Source: CAD feature listing. Evaluate the final solid. Frame: model axes, mm. A direction names the side the tool comes from. Give positions to 0.01 mm unless a question says otherwise; leave off trailing zeros. Write each loop counter-clockwise with the first axis right and the second up, starting at its lowest first coordinate (ties: lowest second). Pieces come first, ordered by that corner, then holes. Notation, with made-up numbers: (-38.75, 72.25) -> (-18.75, 72.25) arc R10 ccw to (-18.75, 91.25) -> close; hole circle Ø10 at (33, -38). An arc over 180 degrees is marked (long way). Answer as a JSON object with one key per item and string values. Group by question number.
Item 1: Section query D-D on y = 3.25. Return the cut outline in (x, z).
Item 2: Section query C-C on x = 0. Return the cut outline in (y, z).
Item 3: Section query A-A on z = 6.25. Return the cut outline in (x, y).
Item 4: Section query B-B on z = 1.75. Return the cut outline in (x, y).
Item 5: First-contact query: pin 1 Ø1 at (y, z) = (3, 6) entering from -X; pin 2 Ø1 at (x, z) = (2.5, 6.5) entering from +Y; pin 3 Ø0.8 at (x, y) = (-5.5, 2.5) entering from +Z. Flat tips, straight axial feed; report the tip coordinate or a pass-through.
Item 6: Ray query, probe 1 along X at (y, z) = (3.75, 5); probe 2 along X at (y, z) = (-3.25, 0.75); probe 3 along Y at (x, z) = (-2.25, 2.5). Return the intervals inside material, ascending. Write a range as from..to.
Item 7: Access query for faces 1 (the face through (3, -4, 6)), 2 (the face through (3, 1.5, 6)), 3 (the face through (5.5, 0.1, 2)). Directions: +Z, -Z, +X, -X, +Y, -Y. A direction counts if a zero-diameter tool reaches every point of the face in a straight line with its end or side. Return the directions, or none.
Item 8: Pull-direction query (Y, two-part tool) for faces 4 (the face through (5, -0.1, 3.6)), 5 (the face through (0, 10, 2)), 6 (the face through (0, 0, 3)); classes: pulls with the +Y half, pulls with the -Y half, needs draft (parallel to the pull), parting line crosses it, or undercut.
Autodesk Inventor part; units mm, degrees
ref_plane "YZ Plane" through (0, 0, 0) normal (1, 0, 0) x (0, 1, 0)
ref_plane "XZ Plane" through (0, 0, 0) normal (0, 1, 0) x (-1, 0, 0)
ref_plane "XY Plane" through (0, 0, 0) normal (0, 0, 1) x (1, 0, 0)
sketch "Sketch1" plane through (0, 0, 0) normal (0, 0, 1) x (1, 0, 0)
  line L0 (-6, -10) -> (6, -10)
  line L1 (6, -10) -> (6, 10)
  line L2 (6, 10) -> (-6, 10)
  line L3 (-6, 10) -> (-6, -10)
  line L4 (-6, -10) -> (6, 10) construction
  line L5 (6, -10) -> (-6, 10) construction
  point P0 (0, 0)
  dimension "d0" = 12
  dimension "d1" = 20
extrude "Extrusion1" add sketch "Sketch1" along normal blind 2
sketch "Sketch2" plane through (0, 0, 2) normal (0, 0, 1) x (1, 0, 0)
  line L0 (-5, -10) -> (5, -10)
  line L1 (5, -10) -> (5, 10)
  line L2 (5, 10) -> (-5, 10)
  line L3 (-5, 10) -> (-5, -10)
  line L4 (-5, -10) -> (5, 10) construction
  line L5 (5, -10) -> (-5, 10) construction
  point P0 (0, 0)
  point P1 (-6, 10)
  dimension "d4" = 10
extrude "Extrusion2" add sketch "Sketch2" along normal blind 2
sketch "Sketch3" plane through (0, 0, 4) normal (0, 0, 1) x (1, 0, 0)
  line L0 (-5, 10) -> (-5, -10)
  line L1 (-5, 4) -> (-1.5, 4)
  line L2 (-1.5, 4) -> (-1.5, 1.5)
  line L3 (-1.5, 1.5) -> (-5, 1.5)
  line L4 (-5, -1.5) -> (-1.5, -1.5)
  line L5 (-1.5, -1.5) -> (-1.5, -4)
  line L6 (-1.5, -4) -> (-5, -4)
  line L7 (5, 10) -> (-5, 10)
  line L8 (-5, -10) -> (5, -10)
  point P0 (0, 0)
  dimension "d7" = 6
  dimension "d8" = 2.5
  dimension "d9" = 6
  dimension "d10" = 2.5
  dimension "d11" = 1.5
extrude "Extrusion3" add sketch "Sketch3" along normal blind 4
mirror "Mirror1" about plane through (0, 0, 0) normal (1, 0, 0) of "Extrusion3"
sketch "Sketch4" plane through (0, 0, 0) normal (0, 0, -1) x (-1, 0, 0)
  line L0 (-3.5, -6.25) -> (3.5, -6.25)
  line L1 (3.5, -6.25) -> (3.5, 6.25)
  line L2 (3.5, 6.25) -> (-3.5, 6.25)
  line L3 (-3.5, 6.25) -> (-3.5, -6.25)
  line L4 (-3.5, -6.25) -> (3.5, 6.25) construction
  line L5 (3.5, -6.25) -> (-3.5, 6.25) construction
  line L6 (-6, 10) -> (6, 10)
  point P0 (0, 0)
  dimension "d14" = 12.5
  dimension "d15" = 3.75
  dimension "d16" = 7
extrude "Extrusion4" cut sketch "Sketch4" against normal blind 3
equation "\"d9\" = d7"
equation "\"d10\" = d8"
properties part number "18"
Worked answers:
{
 "1": {"outline": "(-6, 0) -> (-3.5, 0) -> (-3.5, 3) -> (3.5, 3) -> (3.5, 0) -> (6, 0) -> (6, 2) -> (5, 2) -> (5, 8) -> (1.5, 8) -> (1.5, 4) -> (-1.5, 4) -> (-1.5, 8) -> (-5, 8) -> (-5, 2) -> (-6, 2) -> close"},
 "2": {"outline": "(-10, 0) -> (-6.25, 0) -> (-6.25, 3) -> (6.25, 3) -> (6.25, 0) -> (10, 0) -> (10, 4) -> (-10, 4) -> close"},
 "3": {"outline": "(-5, -4) -> (-1.5, -4) -> (-1.5, -1.5) -> (-5, -1.5) -> close; (-5, 1.5) -> (-1.5, 1.5) -> (-1.5, 4) -> (-5, 4) -> close; (1.5, -4) -> (5, -4) -> (5, -1.5) -> (1.5, -1.5) -> close; (1.5, 1.5) -> (5, 1.5) -> (5, 4) -> (1.5, 4) -> close"},
 "4": {"outline": "(-6, -10) -> (6, -10) -> (6, 10) -> (-6, 10) -> close; hole (-3.5, -6.25) -> (3.5, -6.25) -> (3.5, 6.25) -> (-3.5, 6.25) -> close"},
 "5": {"pin 1": "x = -5", "pin 2": "y = 4", "pin 3": "z = 2"},
 "6": {"probe 1": "-5..-1.5, 1.5..5", "probe 2": "-6..-3.5, 3.5..6", "probe 3": "-10..-6.25, 6.25..10"},
 "7": {"face 1": "+Z, +X, -X, -Y", "face 2": "+Z, +X, -X", "face 3": "+Z, +X, +Y, -Y"},
 "8": {"face 4": "needs draft", "face 5": "pulls with the +Y half", "face 6": "undercut"}
}
